The listing builds one solid part. Answer for the finished solid, in the listing's coordinates (mm). Face numbers are marked on the shaded views. Round coordinates to 2 decimals unless told otherwise and drop trailing zeros. Order: outer loops, then holes, each group sorted by start corner. A loop starts at its lowest first (then second) coordinate and runs counter-clockwise, first axis right, second up. Notation, with made-up numbers: M 28,2 L 35,2 A36 ccw 35,40 Z; hole C 83.25,62.5 d9. An arc over 180 degrees is marked long. Put each result on its own line as item: value. Start each with the question number.
1. The part is cut by section D-D (x = 9). Give the vertices of the cut face in (y, z).
2. Consider line 1 (Y direction, x = -21, z = 0.3); line 2 (X direction, y = -16, z = 1.9); line 3 (X direction, y = -6, z = 3.25). Determine where each line is inside the solid, lowest interval first.
3. The mould has two halves that part along X. Classify the marked faces 1, 2, 3 and 4: +X half, -X half, draft (parallel to the pull), parting line (faces both ways), or undercut.
4. The part is cut by section C-C (x = -22). Give the vertices of the cut face in (y, z), then the cut area to 3 significant figures.
5. The part is cut by section B-B (z = 3.3). Give the vertices of the cut face in (x, y), then the cut area to 3 significant figures.
6. Each of these flat-tipped pins is pushed along its axis until it touches: pin 1 Ø16 at (x, y) = (17.9, -10) entering from +Z; pin 2 Ø1.5 at (y, z) = (4.5, 2) entering from +X; pin 3 Ø1.2 at (x, z) = (-18.5, 1) entering from -Y. Where does it stop, or does it pass through?
7. The part is cut by section A-A (y = -10). Give the vertices of the cut face in (x, z), then the cut area to 3 significant figures.
from build123d import *

# Parameters (mm, degrees)
SKETCH_1_R          = 13.5
EXTRUDE_1_DEPTH     = 4
SKETCH_2_R          = 1.45
CUT_EXTRUDE_1_DEPTH = 50.198239165
FILLET_1_R          = 30
FILLET_2_R          = 3


with BuildPart() as part:
    # 草图1 → 凸台-拉伸1 (new body)
    with BuildSketch(Plane.XY):
        with BuildLine():
            Line((0, 0), (-32.104469832, 0))
            Line((-32.104469832, 0), (-32.104469832, -20))
            Line((-32.104469832, -20), (0, -20))
            ThreePointArc((0, -20), (38.395530168, -10), (0, 0))
        make_face()
        with Locations((17.895530168, -10)):
            Circle(SKETCH_1_R, mode=Mode.SUBTRACT)
    extrude(amount=EXTRUDE_1_DEPTH)

    # 草图2 → 切除-拉伸1 (cut, through all)
    with BuildSketch(Plane.XY.offset(4)):
        with Locations((-22.104469832, -5)):
            Circle(SKETCH_2_R)
        with Locations((-12.104469832, -5)):
            Circle(SKETCH_2_R)
        with Locations((-12.104469832, -15)):
            Circle(SKETCH_2_R)
        with Locations((-22.104469832, -15)):
            Circle(SKETCH_2_R)
    extrude(amount=-CUT_EXTRUDE_1_DEPTH, mode=Mode.SUBTRACT)

    # 圆角1
    fillet_1_edges = [part.edges().sort_by_distance(p)[0] for p in [
        (0, -20, 2),
        (0, 0, 2),
    ]]
    fillet(fillet_1_edges, radius=FILLET_1_R)

    # 圆角2
    fillet_2_edges = [part.edges().sort_by_distance(p)[0] for p in [
        (-32.104469832, -20, 2),
        (-32.104469832, 0, 2),
    ]]
    fillet(fillet_2_edges, radius=FILLET_2_R)


solid = part.part
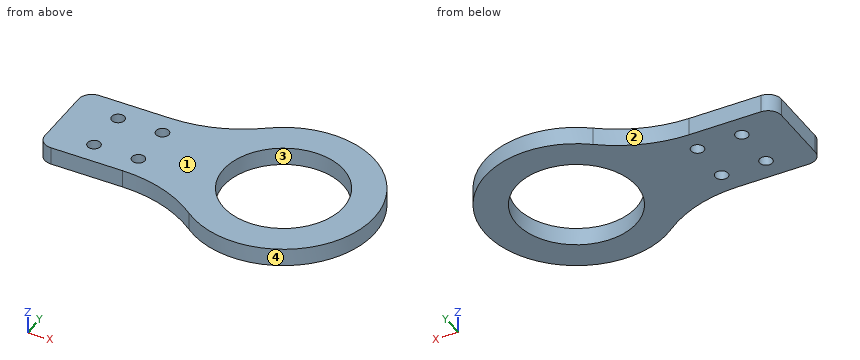
Resolved:
1. outline: M -28.47,0 L -20.15,0 L -20.15,4 L -28.47,4 Z; M 0.15,0 L 8.47,0 L 8.47,4 L 0.15,4 Z
2. line 1: -20 to -15.94, -14.06 to -5.94, -4.06 to 0
2. line 2: -32.1 to -23.15, -21.05 to -13.15, -11.05 to 5.8, 29.99 to 37.5
2. line 3: -32.1 to -23.15, -21.05 to -13.15, -11.05 to 5, 30.79 to 38
3. face 1: draft
3. face 2: -X half
3. face 3: undercut
3. face 4: parting line
4. outline: M -20,0 L -16.45,0 L -16.45,4 L -20,4 Z; M -13.55,0 L -6.45,0 L -6.45,4 L -13.55,4 Z; M -3.55,0 L 0,0 L 0,4 L -3.55,4 Z
4. area: 56.9 mm2
5. outline: M -32.1,-17 A3 ccw -29.1,-20 L -12.93,-20 A30 cw 5.38,-26.24 A20.5 ccw long 5.38,6.24 A30 cw -12.93,0 L -29.1,0 A3 ccw -32.1,-3 Z; hole C -22.1,-15 d2.9; hole C -22.1,-5 d2.9; hole C -12.1,-15 d2.9; hole C -12.1,-5 d2.9; hole C 17.9,-10 d27
5. area: 1,360 mm2
6. pin 1: through
6. pin 2: x = 33.1
6. pin 3: y = -20
7. outline: M -32.1,0 L 4.4,0 L 4.4,4 L -32.1,4 Z; M 31.4,0 L 38.4,0 L 38.4,4 L 31.4,4 Z
7. area: 174 mm2
